```python
from build123d import *

# Parameters (mm, degrees)
SKETCH_1_W          = 85
SKETCH_1_H          = 85
EXTRUDE_1_DEPTH     = 2
SKETCH_2_R          = 9
CUT_EXTRUDE_1_DEPTH = 2
SKETCH_3_R          = 5
CUT_EXTRUDE_3_DEPTH = 1
SKETCH_4_R          = 5
CUT_EXTRUDE_4_DEPTH = 1
SKETCH_5_R          = 1
CUT_EXTRUDE_5_DEPTH = 94.644624303
CHAMFER_1_SIZE      = 1
CHAMFER_2_SIZE      = 1


with BuildPart() as part:
    # 草图1 → 凸台-拉伸1 (new body)
    with BuildSketch(Plane.XY):
        with Locations((27.114602804, -20.102897196)):
            Rectangle(SKETCH_1_W, SKETCH_1_H)
    extrude(amount=EXTRUDE_1_DEPTH)

    # 草图2 → 切除-拉伸1 (cut)
    with BuildSketch(Plane(origin=(0, 0, 0), x_dir=(-1, 0, 0), z_dir=(0, 0, -1))):
        with Locations((-27.114602804, -20.102897196)):
            Circle(SKETCH_2_R)
    extrude(amount=-CUT_EXTRUDE_1_DEPTH, mode=Mode.SUBTRACT)

    # 草图3 → 切除-拉伸3 (cut)
    with BuildSketch(Plane.XY.offset(2)):
        with Locations((49.614602804, -20.495049302)):
            Circle(SKETCH_3_R)
        with Locations((27.114602804, 2.397102804)):
            Circle(SKETCH_3_R)
        with Locations((27.114602804, -42.995049302)):
            Circle(SKETCH_3_R)
        with Locations((4.614602804, -20.102897196)):
            Circle(SKETCH_3_R)
    extrude(amount=-CUT_EXTRUDE_3_DEPTH, mode=Mode.SUBTRACT)

    # 草图4 → 切除-拉伸4 (cut)
    with BuildSketch(Plane(origin=(0, 0, 0), x_dir=(-1, 0, 0), z_dir=(0, 0, -1))):
        with Locations((-49.215493554, -42.995049302)):
            Circle(SKETCH_4_R)
        with Locations((-38.165048179, -31.548973249)):
            Circle(SKETCH_4_R)
        with Locations((-49.614602804, 2.397102804)):
            Circle(SKETCH_4_R)
        with Locations((-38.364602804, -8.852897196)):
            Circle(SKETCH_4_R)
        with Locations((-4.614602804, -42.602897196)):
            Circle(SKETCH_4_R)
        with Locations((-15.864602804, -31.352897196)):
            Circle(SKETCH_4_R)
        with Locations((-4.614602804, 2.397102804)):
            Circle(SKETCH_4_R)
        with Locations((-15.864602804, -8.852897196)):
            Circle(SKETCH_4_R)
    extrude(amount=-CUT_EXTRUDE_4_DEPTH, mode=Mode.SUBTRACT)

    # 草图5 → 切除-拉伸5 (cut, through all)
    with BuildSketch(Plane(origin=(0, 0, 0), x_dir=(-1, 0, 0), z_dir=(0, 0, -1))):
        with Locations((-4.614602804, -42.602897196)):
            Circle(SKETCH_5_R)
        with Locations((-15.864602804, -31.352897196)):
            Circle(SKETCH_5_R)
        with Locations((-15.864602804, -8.852897196)):
            Circle(SKETCH_5_R)
        with Locations((-4.614602804, 2.397102804)):
            Circle(SKETCH_5_R)
        with Locations((-38.364602804, -8.852897196)):
            Circle(SKETCH_5_R)
        with Locations((-49.614602804, 2.397102804)):
            Circle(SKETCH_5_R)
        with Locations((-49.215493554, -42.995049302)):
            Circle(SKETCH_5_R)
        with Locations((-38.165048179, -31.548973249)):
            Circle(SKETCH_5_R)
    extrude(amount=-CUT_EXTRUDE_5_DEPTH, mode=Mode.SUBTRACT)

    # 倒角1
    chamfer_1_edges = [part.edges().sort_by_distance(p)[0] for p in [
        (36.114602804, -20.102897196, 0),
    ]]
    chamfer(chamfer_1_edges, length=CHAMFER_1_SIZE)

    # 倒角2
    chamfer_2_edges = [part.edges().sort_by_distance(p)[0] for p in [
        (36.114602804, -20.102897196, 2),
    ]]
    chamfer(chamfer_2_edges, length=CHAMFER_2_SIZE - 0.0001)  # a hair under: the kernel refuses the full size

    # 圆角1: read off the stored shape, not the designer's step
    # 圆角1 outline → 圆角1 (revolve, cut)
    with BuildSketch(Plane(origin=(27.114602804, -20.102897196, 0), x_dir=(1, 0, 0), z_dir=(0, -1, 0))):
        with BuildLine():
            ThreePointArc((9.707106781, 0.292893219), (9.414213562, 1), (9.707106781, 1.707106781))
            Line((9.707106781, 1.707106781), (0, 1.707106781))
            Line((0, 1.707106781), (0, 0.292893219))
            Line((0, 0.292893219), (9.707106781, 0.292893219))
        make_face()
    revolve(axis=Axis((27.114602804, -20.102897196, 0), (0, 0, 1)), mode=Mode.SUBTRACT)


solid = part.part
```
Input: part model. Units: mm. Frame: model coordinates. A direction names the side the tool comes from. Give positions to 0.01 mm unless a question says otherwise; leave off trailing zeros.
1. Line query: probe 1 along X at (y, z) = (-21, 1.1); probe 2 along Y at (x, z) = (16, 1.7); probe 3 along Y at (x, z) = (39, 0.4). Output: solid intervals per line, ascending.
Computed:
probe 1: x = -15.39 to -0.3, 9.53 to 17.74, 36.49 to 44.64, 54.59 to 69.61
probe 2: y = -62.6 to -32.34, -30.36 to -9.84, -7.86 to 22.4
probe 3: y = -62.6 to -36.48, -26.62 to -13.81, -3.89 to 22.4
2. Set-up query: faces 1 (the face through (14.91, -8.55, 1.49)), 2 (the face through (48, -43, 1)), 3 (the face through (52.303, -16.279, 1.507)). Return all of +Z, -Z, +X, -X, +Y, -Y with unobstructed straight access to the full face (end or side cutting, diameter ignored); none if empty.
Computed:
face 1: +Z, -Z
face 2: -Z
face 3: +Z
3. Pin query (flat end, axial travel): pin 1 Ø5 at (x, y) = (39.5, -7.5) entering from -Z; pin 2 Ø8 at (x, y) = (3.5, -19.5) entering from +Z; pin 3 Ø9 at (x, y) = (4.61, -20.1) entering from +Z. Return the tip coordinate at first contact, or that it passes through.
Computed:
pin 1: stops at z = 1
pin 2: stops at z = 2
pin 3: stops at z = 1
4. Draft query along Y for faces 4 (the face through (27, -38, 0)), 5 (the face through (53.18, -46.04, 0.49)), 6 (the face through (27, -62.603, 1)). Return one class per face: released by +Y, released by -Y, zero draft, split by the parting line, or undercut.
Computed:
face 4: zero draft
face 5: undercut
face 6: released by -Y
